from build123d import *

# Parameters (mm, degrees)
BASPROSKE_W           = 4
BASPROSKE_H           = 5
TOOTHCUT_DEPTH        = 9.124038405
TEETHCUTS_COUNT       = 18
TEETHCUTS_ANGLE       = 340
BORSKE_R              = 1
BORE_DEPTH            = 50.0000508
BODY_MOVE_COPY1_ANGLE = 90
BODY_MOVE_COPY2_ANGLE = 90


with BuildPart() as part:
    # BasProSke → Base-Revolve (revolve)
    with BuildSketch(Plane(origin=(0, 0, 0), x_dir=(1, 0, 0), z_dir=(0, 1, 0)), mode=Mode.PRIVATE) as base_revolve_sk:
        with Locations((2, 2.5)):
            Rectangle(BASPROSKE_W, BASPROSKE_H)
    revolve(base_revolve_sk.sketch.rotate(Axis((-10, 0, 0), (1, 0, 0)), 180), axis=Axis((-10, 0, 0), (1, 0, 0)))

    # TooCutSke → ToothCut (cut, through all)
    with BuildSketch(Plane(origin=(0, 0, 0), x_dir=(0, 0, -1), z_dir=(1, 0, 0))):
        with BuildLine():
            ThreePointArc((0.25527463, 3.865580275), (0, 3.874), (-0.25527463, 3.865580275))
            ThreePointArc((-0.25527463, 3.865580275), (-0.416281865, 4.46052923), (-0.768562654, 4.96628197))
            ThreePointArc((-0.768562654, 4.96628197), (0, 5.0254), (0.768562654, 4.96628197))
            ThreePointArc((0.768562654, 4.96628197), (0.416281865, 4.46052923), (0.25527463, 3.865580275))
        make_face()
    toothcut = extrude(amount=TOOTHCUT_DEPTH, mode=Mode.SUBTRACT)

    # TeethCuts: ToothCut ×18 about axis
    teethcuts_axis = Axis((-10, 0, 0), (1, 0, 0))
    for i in range(1, TEETHCUTS_COUNT):
        add(toothcut.rotate(teethcuts_axis, i * TEETHCUTS_ANGLE / (TEETHCUTS_COUNT - 1)), mode=Mode.SUBTRACT)

    # BorSke → Bore (cut, symmetric)
    with BuildSketch(Plane(origin=(0, 0, 0), x_dir=(0, 0, -1), z_dir=(1, 0, 0))):
        with Locations(Location((0, 0, 0), (0, 0, 180))):
            Circle(BORSKE_R)
    extrude(amount=BORE_DEPTH, both=True, mode=Mode.SUBTRACT)


with BuildPart() as part_1:
    # Body-Move/Copy1: moved
    add(part.part.rotate(Axis((2, 0, 0), (0, 0, -1)), BODY_MOVE_COPY1_ANGLE))


with BuildPart() as part_2:
    # Body-Move/Copy2: moved
    add(part_1.part.rotate(Axis((0, 0, 0), (-1, 0, 0)), BODY_MOVE_COPY2_ANGLE))


solid = part_2.part
For this review, take the finished solid that the model builds, in its own axes (mm). A direction names the side the tool comes from. Give positions to 0.01 mm unless a question says otherwise; leave off trailing zeros. Loops run counter-clockwise (first coordinate to the right, second up) from the corner with the lowest first, then second, coordinate; pieces in that order, holes last.
Item 1: Take a section at C-C, the plane y = 4.5. State the section outline as (x, z) points.
Item 2: Draft analysis for pull direction X (two halves, no side actions). For faces 1 (the cylindrical face through (2.37, 4.44, -0.03)), 2 (the cylindrical face through (5.139, 3.164, -0.028)), 3 (the flat face through (1.9, 1.2, -2)), state which applies: +X half, -X half, draft (parallel to the pull), parting line (faces both ways), or undercut.
Item 3: Insertion check: pin 1 (2 mm diameter, centred on y = -3, z = 1, fed in from -X); pin 2 (1 mm diameter, centred on y = -3.5, z = -0.5, fed in from +X); pin 3 (2.5 mm diameter, centred on x = 2, y = 0, fed in from -Z). Each pin has a flat end and moves straight along its axis. Give the tip position at first contact, or say it passes through.
Item 4: For line 1 along X through (y, z) = (0, 0.8); line 2 along Y through (x, z) = (6, -0.5); line 3 along Y through (x, z) = (2, -0.9), list the stretches that pass through material, from the lowest coordinate up.
Item 5: Take a section at B-B, the plane x = 2. State the section outline as (y, z) points.
Item 6: Tool access review of faces 4 (the cylindrical face through (5.678, 2.546, -0.028)), 5 (the cylindrical face through (-2.03, -1.9, -0.03)), 6 (the cylindrical face through (0.82, -4.315, -0.028)), 7 (the cylindrical face through (5.146, -3.18, -0.028)): name each direction out of +Z, -Z, +X, -X, +Y, -Y from which nothing blocks a thin tool from reaching the whole face with its end or side.
Item 7: Take a section at A-A, the plane y = 0. State the section outline as (x, z) points.
Calculated:
1. outline: (0.14, -2) - (0.67, -2) - (0.67, 2) - (0.14, 2) - close; (1.65, -2) - (2.35, -2) - (2.35, 2) - (1.65, 2) - close; (3.33, -2) - (3.86, -2) - (3.86, 2) - (3.33, 2) - close
2. face 1: undercut
2. face 2: +X half
2. face 3: draft
3. pin 1: stops at x = -2.39
3. pin 2: stops at x = 5.31
3. pin 3: stops at z = -2
4. line 1: x = -1.87 to 1, 3 to 5.87
4. line 2: y = -2.6 to -1.87, -1.13 to -0.27, 0.27 to 1.13, 1.87 to 2.6
4. line 3: y = -5 to -1, 1 to 5
5. outline: (-5, -2) - (-1, -2) - (-1, 2) - (-5, 2) - close; (1, -2) - (5, -2) - (5, 2) - (1, 2) - close
6. face 4: +Z, -Z
6. face 5: +Z, -Z, -X
6. face 6: +Z, -Z, -Y
6. face 7: +Z, -Z, +X
7. outline: (-1.87, -2) - (1, -2) - (1, 2) - (-1.87, 2) - close; (3, -2) - (5.87, -2) - (5.87, 2) - (3, 2) - close
